```python
from build123d import *

# Parameters (mm, degrees)
BASE_EXTRUDE_DEPTH = 90
SKETCH2_R          = 15
CUT_EXTRUDE1_DEPTH = 94.841621896
SKETCH3_R          = 6
CUT_EXTRUDE2_DEPTH = 100.058063781
FILLET1_R          = 6


with BuildPart() as part:
    # Sketch1 → Base-Extrude (new body)
    with BuildSketch(Plane.XY):
        with BuildLine():
            Line((-17.5, -20), (-17.5, 0))
            ThreePointArc((-17.5, 0), (0, 17.5), (17.5, 0))
            Line((17.5, 0), (17.5, -20))
            Line((17.5, -20), (-17.5, -20))
        make_face()
    extrude(amount=BASE_EXTRUDE_DEPTH)

    # Sketch2 → Cut-Extrude1 (cut, through all)
    with BuildSketch(Plane.XY.offset(90)):
        Circle(SKETCH2_R)
    extrude(amount=-CUT_EXTRUDE1_DEPTH, mode=Mode.SUBTRACT)

    # Sketch3 → Cut-Extrude2 (cut, through all)
    with BuildSketch(Plane.XZ.offset(20)):
        with Locations((0, 35)):
            Circle(SKETCH3_R)
        with Locations((0, 75)):
            Circle(SKETCH3_R)
    extrude(amount=-CUT_EXTRUDE2_DEPTH, mode=Mode.SUBTRACT)

    # Fillet1
    fillet1_edges = [part.edges().sort_by_distance(p)[0] for p in [
        (17.5, -20, 45),
        (-17.5, -20, 45),
    ]]
    fillet(fillet1_edges, radius=FILLET1_R)


solid = part.part
```
Verification items for the finished model (mm, model axes). Give positions to 0.01 mm unless a question says otherwise; leave off trailing zeros. Write each loop counter-clockwise with the first axis right and the second up, starting at its lowest first coordinate (ties: lowest second). Pieces come first, ordered by that corner, then holes. Notation, with made-up numbers: (86.25, 27) - (104.25, 27) arc R28 ccw to (104.25, 53) - close; hole circle Ø7 at (50, -26). An arc over 180 degrees is marked (long way). Put each result on its own line as item: value.
Q1. Section check B-B on z = 35. Record the cut outline in (x, y).
Result:
outline: (-17.5, -14) arc R6 ccw to (-11.5, -20) - (-6, -20) - (-6, -13.75) arc R15 cw to (-6, 13.75) - (-6, 16.44) arc R17.5 ccw to (-17.5, 0) - close; (6, -20) - (11.5, -20) arc R6 ccw to (17.5, -14) - (17.5, 0) arc R17.5 ccw to (6, 16.44) - (6, 13.75) arc R15 cw to (6, -13.75) - close
Q2. Section check A-A on x = 0. Record the cut outline in (y, z), and give its area (3 significant figures).
Result:
outline: (-20, 0) - (-15, 0) - (-15, 29) - (-20, 29) - close; (-20, 41) - (-15, 41) - (-15, 69) - (-20, 69) - close; (-20, 81) - (-15, 81) - (-15, 90) - (-20, 90) - close; (15, 0) - (17.5, 0) - (17.5, 29) - (15, 29) - close; (15, 41) - (17.5, 41) - (17.5, 69) - (15, 69) - close; (15, 81) - (17.5, 81) - (17.5, 90) - (15, 90) - close
area: 495 mm2
Q3. Section check D-D on y = 4.5. Record the cut outline in (x, z), and give its area (3 significant figures).
Result:
outline: (-16.91, 0) - (-14.31, 0) - (-14.31, 90) - (-16.91, 90) - close; (14.31, 0) - (16.91, 0) - (16.91, 90) - (14.31, 90) - close
area: 468 mm2
Q4. Mould release check, pull along Y, two halves, no side actions. Record for faces 1 (the face through (-15.789, -18.196, 45.63)), 2 (the face through (14.307, 4.506, 45.63)), 3 (the face through (8, -13, 90)): released by +Y, released by -Y, zero draft, split by the parting line, or undercut.
Result:
face 1: released by -Y
face 2: undercut
face 3: zero draft
Q5. Section check C-C on z = 51. Record the cut outline in (x, y).
Result:
outline: (-17.5, -14) arc R6 ccw to (-11.5, -20) - (11.5, -20) arc R6 ccw to (17.5, -14) - (17.5, 0) arc R17.5 ccw to (-17.5, 0) - close; hole circle Ø30 at (0, 0)
Q6. Scan lines: probe 1 along Z at (x, y) = (0, -17); probe 2 along Z at (x, y) = (-4, -18); probe 3 along Y at (x, z) = (0, 22.5). Record each from-to range of solid material in increasing order. Write a range as from..to.
Result:
probe 1: 0..29, 41..69, 81..90
probe 2: 0..30.53, 39.47..70.53, 79.47..90
probe 3: -20..-15, 15..17.5
Q7. Depth check by flat-ended pin: P1, Ø11, axis at x = 0, z = 35, coming from the +Y side; P2, Ø3, axis at x = 11, z = 54, coming from the +Y side; P3, Ø5, axis at x = 13.5, z = 73.5, coming from the +Y side; P4, Ø3, axis at y = 9, z = 68, coming from the +X side. Enter the tip coordinate at first touch or a pass-through.
Result:
P1: through
P2: y = 14.7
P3: y = 13.61
P4: x = 15.81
